from build123d import *

# Parameters (mm, degrees)
SKETCH_1_W          = 96
SKETCH_1_H          = 145
EXTRUDE_1_DEPTH     = 2
SKETCH_2_W          = 6.362526911
SKETCH_2_H          = 29.426686961
SKETCH_2_H_2        = 22.799054763
SKETCH_2_H_3        = 9.808895654
SKETCH_2_H_4        = 10.869316806
SKETCH_2_H_5        = 27.04073937
EXTRUDE_2_DEPTH     = 17
SKETCH_3_W          = 29.426686961
SKETCH_3_H          = 17.496949003
EXTRUDE_3_DEPTH     = 46
SKETCH_4_W          = 9.808895653
SKETCH_4_H          = 22.268844187
SKETCH_4_W_2        = 10.33910623
SKETCH_4_W_3        = 9.676343009
SKETCH_4_H_2        = 26.510528793
EXTRUDE_4_DEPTH     = 25
SKETCH_5_R          = 5.037000471
EXTRUDE_5_DEPTH     = 10
SKETCH_6_W          = 7.157842775
SKETCH_6_H          = 16.70163314
EXTRUDE_6_DEPTH     = 10
SKETCH_7_W          = 7.157842774
SKETCH_7_H          = 73.699270047
SKETCH_7_W_2        = 7.68805335
EXTRUDE_7_DEPTH     = 10
SKETCH_8_R          = 1.6
CUT_EXTRUDE_1_DEPTH = 99.367931766
SKETCH_9_W          = 70
SKETCH_9_H          = 10
EXTRUDE_8_DEPTH     = 10.5
SKETCH_10_W         = 70
SKETCH_10_H         = 2.5
EXTRUDE_9_DEPTH     = 2
EXTRUDE_10_DEPTH    = 8
SKETCH_12_R         = 2.5
EXTRUDE_11_DEPTH    = 6
M3X0_5_1_D          = 2.5
M3X0_5_1_DEPTH      = 7.5
M3X0_5_1_TIP        = 0.751075774


with BuildPart() as part:
    # 草图1 → 凸台-拉伸1 (new body)
    with BuildSketch(Plane.XY):
        Rectangle(SKETCH_1_W, SKETCH_1_H)
    extrude(amount=EXTRUDE_1_DEPTH)

    # 草图2 → 凸台-拉伸2 (add)
    with BuildSketch(Plane.XY.offset(2)):
        with Locations((-40.296003767, 52.7559523)):
            Rectangle(SKETCH_2_W, SKETCH_2_H)
        with Locations((-40.296003767, 18.159712224)):
            Rectangle(SKETCH_2_W, SKETCH_2_H_2)
        with Locations((-40.296003767, -9.543790366)):
            Rectangle(SKETCH_2_W, SKETCH_2_H_3)
        with Locations((-40.296003767, -29.161581673)):
            Rectangle(SKETCH_2_W, SKETCH_2_H_4)
        with Locations((-40.296003767, -53.418715519)):
            Rectangle(SKETCH_2_W, SKETCH_2_H_5)
    extrude(amount=EXTRUDE_2_DEPTH)

    # 草图3 → 凸台-拉伸3 (add)
    with BuildSketch(Plane.XY.offset(2)):
        with Locations((-17.364396359, 52.09318908)):
            Rectangle(SKETCH_3_W, SKETCH_3_H)
    extrude(amount=EXTRUDE_3_DEPTH)

    # 草图4 → 凸台-拉伸4 (add)
    with BuildSketch(Plane.XY.offset(2)):
        with Locations((-22.931607407, 18.159712224)):
            Rectangle(SKETCH_4_W, SKETCH_4_H)
        with Locations((-8.085711282, 18.159712224)):
            Rectangle(SKETCH_4_W_2, SKETCH_4_H)
        with Locations((-18.093435902, -22.401396831)):
            Rectangle(SKETCH_4_W_3, SKETCH_4_H_2)
    extrude(amount=EXTRUDE_4_DEPTH)

    # 草图5 → 凸台-拉伸5 (add)
    with BuildSketch(Plane.XY.offset(2)):
        with Locations((-13.520369685, -46.791083321)):
            Circle(SKETCH_5_R)
    extrude(amount=EXTRUDE_5_DEPTH)

    # 草图6 → 凸台-拉伸6 (add)
    with BuildSketch(Plane.XY.offset(2)):
        with Locations((22.666502119, 53.286162875)):
            Rectangle(SKETCH_6_W, SKETCH_6_H)
    extrude(amount=EXTRUDE_6_DEPTH)

    # 草图7 → 凸台-拉伸7 (add)
    with BuildSketch(Plane.XY.offset(2)):
        with Locations((21.075870391, -11.00186945)):
            Rectangle(SKETCH_7_W, SKETCH_7_H)
        with Locations((36.982187667, -11.00186945)):
            Rectangle(SKETCH_7_W_2, SKETCH_7_H)
    extrude(amount=EXTRUDE_7_DEPTH)

    # 草图8 → 切除-拉伸1 (cut, through all)
    with BuildSketch(Plane.XY.offset(2)):
        with Locations((-31.5, -51.5)):
            Circle(SKETCH_8_R)
        with Locations((28.5, -51.5)):
            Circle(SKETCH_8_R)
        with Locations((-31.5, 38.5)):
            Circle(SKETCH_8_R)
        with Locations((28.5, 38.5)):
            Circle(SKETCH_8_R)
    extrude(amount=-CUT_EXTRUDE_1_DEPTH, mode=Mode.SUBTRACT)

    # 草图9 → 凸台-拉伸8 (add)
    with BuildSketch(Plane.XY.offset(2)):
        with Locations((2, -67.5)):
            Rectangle(SKETCH_9_W, SKETCH_9_H)
    extrude(amount=EXTRUDE_8_DEPTH)

    # 草图10 → 凸台-拉伸9 (add)
    with BuildSketch(Plane.XY.offset(12.5)):
        with Locations((2, -71.25)):
            Rectangle(SKETCH_10_W, SKETCH_10_H)
    extrude(amount=EXTRUDE_9_DEPTH)

    # 草图11 → 凸台-拉伸10 (add)
    with BuildSketch(Plane.XZ.offset(72.5)):
        Polygon((-25, 12.175), (29, 12.175), (27.5, 4.325), (-23.5, 4.325), align=None)
    extrude(amount=EXTRUDE_10_DEPTH)

    # 草图12 → 凸台-拉伸11 (add)
    with BuildSketch(Plane.XZ.offset(72.5)):
        with Locations(Location((-29.75, 8.25, 0), (0, 0, 90))):
            Circle(SKETCH_12_R)
        with Locations(Location((33.75, 8.25, 0), (0, 0, 90))):
            Circle(SKETCH_12_R)
    extrude(amount=EXTRUDE_11_DEPTH)

    # M3x0.5 螺纹孔1
    with Locations(Plane.XZ.offset(78.5)):
        with Locations((-29.75, 8.25), (33.75, 8.25)):
            Hole(M3X0_5_1_D / 2, depth=M3X0_5_1_DEPTH)
            with Locations((0, 0, -(M3X0_5_1_DEPTH + M3X0_5_1_TIP / 2))):  # 118° drill point
                Cone(0, M3X0_5_1_D / 2, M3X0_5_1_TIP, mode=Mode.SUBTRACT)


solid = part.part
Geometry: final body of the model. Coordinates: model frame, mm. A direction names the side the tool comes from. Coordinates: 2 decimals unless noted, no trailing zeros. Order: outer loops, then holes, each group sorted by start corner. A loop starts at its lowest first (then second) coordinate and runs counter-clockwise, first axis right, second up.
(1) Access query for faces 1 (the face through (-13.255, 18, 14)), 2 (the face through (-40, 67.469, 10)), 3 (the face through (37, -10, 12)). Directions: +Z, -Z, +X, -X, +Y, -Y. A direction counts if a zero-diameter tool reaches every point of the face in a straight line with its end or side. Return the directions, or none.
(2) First-contact query: pin 1 (2.5 mm diameter, centred on x = 4, y = -77, fed in from +Z) (3 decimals); pin 2 (8 mm diameter, centred on x = -23, z = 38, fed in from +Y); pin 3 (5 mm diameter, centred on x = 18.5, y = 27.5, fed in from +Z); pin 4 (12 mm diameter, centred on x = 31, z = 25, fed in from +Y). Flat tips, straight axial feed; report the tip coordinate or a pass-through.
(3) Section query B-B (z = 44.5). Return the cut outline in (x, y), plus the area to 3 significant figures.
(4) Material intervals for probe 1 along X at (y, z) = (53, 4); probe 2 along Y at (x, z) = (-31.5, 1.3); probe 3 along Y at (x, z) = (-23, 4.5), sorted ascending.
(5) Section query A-A (x = 15). Return the cut outline in (y, z) (3 decimals), plus the area to 3 significant figures.
(6) Section query D-D (x = -15.5). Return the cut outline in (y, z) (3 decimals), plus the area to 3 significant figures.
(7) Section query C-C (x = 39). Return the cut outline in (y, z).
Solution:
1. face 1: +Z
1. face 2: +Z, +X, -X, +Y
1. face 3: +Z, +X, +Y
2. pin 1: stops at z = 12.175
2. pin 2: stops at y = 60.84
2. pin 3: stops at z = 12
2. pin 4: passes through
3. outline: (-32.08, 43.34) - (-2.65, 43.34) - (-2.65, 60.84) - (-32.08, 60.84) - close
3. area: 515 mm2
4. probe 1: x = -43.48 to -37.11, -32.08 to -2.65, 19.09 to 26.25
4. probe 2: y = -72.5 to -53.1, -49.9 to 36.9, 40.1 to 72.5
4. probe 3: y = -80.5 to -62.5, 7.03 to 29.29, 43.34 to 60.84
5. outline: (-80.5, 4.325) - (-72.5, 4.325) - (-72.5, 0) - (72.5, 0) - (72.5, 2) - (-62.5, 2) - (-62.5, 12.5) - (-70, 12.5) - (-70, 14.5) - (-72.5, 14.5) - (-72.5, 12.175) - (-80.5, 12.175) - close
5. area: 463 mm2
6. outline: (-80.5, 4.325) - (-72.5, 4.325) - (-72.5, 0) - (72.5, 0) - (72.5, 2) - (60.842, 2) - (60.842, 48) - (43.345, 48) - (43.345, 2) - (-9.146, 2) - (-9.146, 27) - (-35.657, 27) - (-35.657, 2) - (-42.159, 2) - (-42.159, 12) - (-51.423, 12) - (-51.423, 2) - (-62.5, 2) - (-62.5, 12.5) - (-70, 12.5) - (-70, 14.5) - (-72.5, 14.5) - (-72.5, 12.175) - (-80.5, 12.175) - close
6. area: 2,020 mm2
7. outline: (-72.5, 0) - (72.5, 0) - (72.5, 2) - (25.85, 2) - (25.85, 12) - (-47.85, 12) - (-47.85, 2) - (-72.5, 2) - close
